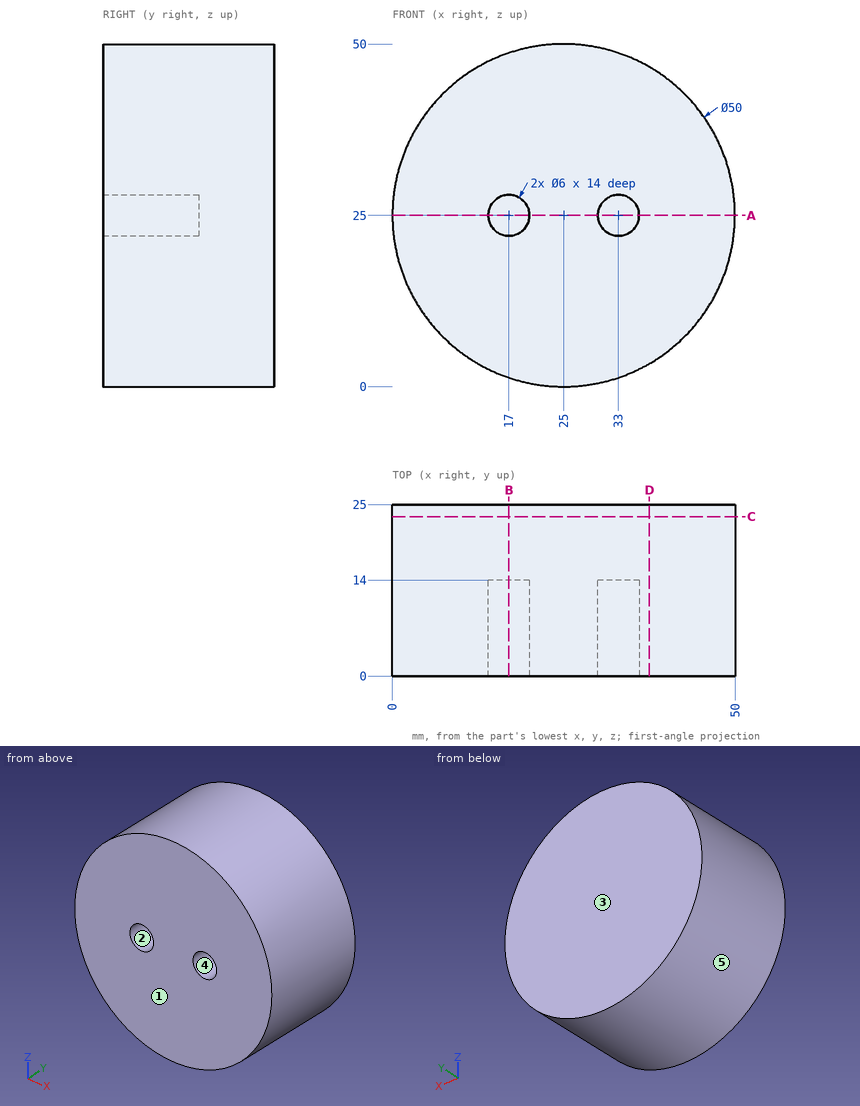
Geometry: see drawing. Coordinates: mm, zero at the bounding-box minimum. A direction names the side the tool comes from. Round coordinates to 2 decimals unless told otherwise and drop trailing zeros. Write each loop counter-clockwise with the first axis right and the second up, starting at its lowest first coordinate (ties: lowest second). Pieces come first, ordered by that corner, then holes. Notation, with made-up numbers: M -4.5,78.5 L 26.5,78.5 A28 ccw 26.5,115.5 Z; hole C 32,32 d7. An arc over 180 degrees is marked long. Answer as a JSON object with one key per item and string values. Group by question number.
(1) Section query D-D on x = 37.5. Output: boundary loops of the cut face in (y, z).
(2) First-contact query: pin 1 (10 mm diameter, centred on y = 4, z = 11.5, fed in from +X); pin 2 (10 mm diameter, centred on y = 7.5, z = 14, fed in from +X); pin 3 (5 mm diameter, centred on x = 33.5, z = 24.5, fed in from -Y); pin 4 (6 mm diameter, centred on y = 10, z = 15.5, fed in from +X). Flat tips, straight axial feed; report the tip coordinate or a pass-through.
(3) Section query A-A on z = 25. Output: boundary loops of the cut face in (x, y).
(4) Section query C-C on y = 23.25. Output: boundary loops of the cut face in (x, z), then the cut area to 3 significant figures.
(5) Reachability of the marked faces 1 and 2 from +Z, -Z, +X, -X, +Y, -Y: full face, straight path, thin tool, end or side. Return the list, or none.
(6) Section query B-B on x = 17. Output: boundary loops of the cut face in (y, z), then the cut area to 3 significant figures.
(7) Ray query, line 1 (Z direction, x = 17, y = 5); line 2 (Z direction, x = 33.5, y = 6.5); line 3 (Z direction, x = 46, y = 17.5). Return the intervals inside material, ascending. Write a range as [from, to].
(8) Mould query, pull axis Z, two halves, no side actions, for the marked faces 3, 4 and 5. Classes: +Z half, -Z half, draft (parallel to the pull), parting line (faces both ways), or undercut.
Computed values:
{
 "1": {"outline": "M 0,3.35 L 25,3.35 L 25,46.65 L 0,46.65 Z"},
 "2": {"pin 1": "x = 48.51", "pin 2": "x = 49.27", "pin 3": "y = 0", "pin 4": "x = 49.14"},
 "3": {"outline": "M 0,0 L 14,0 L 14,14 L 20,14 L 20,0 L 30,0 L 30,14 L 36,14 L 36,0 L 50,0 L 50,25 L 0,25 Z"},
 "4": {"outline": "C 25,25 d50", "area": "1,960 mm^2"},
 "5": {"face 1": "+Z, -Z, +X, -X, -Y", "face 2": "-Y"},
 "6": {"outline": "M 0,1.31 L 25,1.31 L 25,48.69 L 0,48.69 L 0,28 L 14,28 L 14,22 L 0,22 Z", "area": "1,100 mm^2"},
 "7": {"line 1": "[1.31, 22], [28, 48.69]", "line 2": "[1.49, 22.04], [27.96, 48.51]", "line 3": "[11.44, 38.56]"},
 "8": {"face 3": "draft", "face 4": "undercut", "face 5": "parting line"}
}
